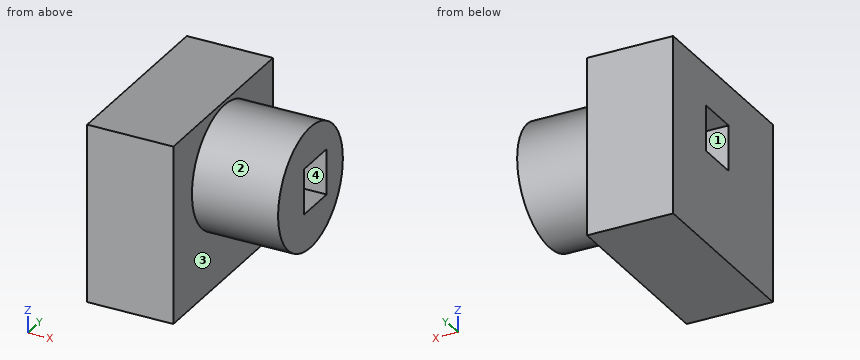
```python
from build123d import *

# Parameters (mm, degrees)
F0_W     = 54.889154
F0_H     = 52.407466
F1_DEPTH = 25.4
F2_R     = 17.820704
F3_DEPTH = 25.4
F4_W     = 12.562469
F4_H     = 13.418828
F5_DEPTH = 50.801


with BuildPart() as f1:
    # F0 (on Right) → F1 (new body)
    with BuildSketch(Plane.YZ):
        with Locations((27.444577, -26.203733)):
            Rectangle(F0_W, F0_H)
    extrude(amount=F1_DEPTH)

    # F2 (on face) → F3 (join)
    with BuildSketch(Plane.YZ.offset(25.4)):
        with Locations((28.055245, -18.92175)):
            Circle(F2_R)
    extrude(amount=F3_DEPTH)

    # F4 (on face) → F5 (cut, through all)
    with BuildSketch(Plane.YZ.offset(50.8)):
        with Locations((30.671432, -18.585598)):
            Rectangle(F4_W, F4_H)
    extrude(amount=-F5_DEPTH, mode=Mode.SUBTRACT)


solid = f1.part
```
Input: part model. Units: mm. Frame: model coordinates. Face numbers are marked on the shaded views. Round coordinates to 2 decimals unless told otherwise and drop trailing zeros. Order: outer loops, then holes, each group sorted by start corner. A loop starts at its lowest first (then second) coordinate and runs counter-clockwise, first axis right, second up. Notation, with made-up numbers: (34, 40.5) - (85, 40.5) arc R23 cw to (85, 77.5) - close; hole circle Ø11 at (45, 57). An arc over 180 degrees is marked (long way). Answer in a Markdown table with one row per item.
Item 1: Section query D-D (z = -34.5). Return the cut outline in (x, y).
Model answer:
| item | result |
|---|---|
| outline | (0, 0) - (25.4, 0) - (25.4, 19.4) - (50.8, 19.4) - (50.8, 36.71) - (25.4, 36.71) - (25.4, 54.89) - (0, 54.89) - close |
Item 2: Pin query (flat end, axial travel): pin 1 (1.5 mm diameter, centred on y = 16, z = -42.5, fed in from +X); pin 2 (10 mm diameter, centred on x = 16, y = 13.5, fed in from +Z); pin 3 (1 mm diameter, centred on x = 36.5, y = 27.5, fed in from -Z); pin 4 (6 mm diameter, centred on x = 40.5, y = 12.5, fed in from +Z). Return the tip coordinate at first contact, or that it passes through.
Model answer:
| item | result |
|---|---|
| pin 1 | stops at x = 25.4 |
| pin 2 | stops at z = 0 |
| pin 3 | stops at z = -36.74 |
| pin 4 | stops at z = -6.27 |
Item 3: Section query A-A (x = 22). Return the cut outline in (y, z), then the cut area to 3 significant figures.
Model answer:
| item | result |
|---|---|
| outline | (0, -52.41) - (54.89, -52.41) - (54.89, 0) - (0, 0) - close; hole (24.39, -25.3) - (36.95, -25.3) - (36.95, -11.88) - (24.39, -11.88) - close |
| area | 2,710 mm² |
Item 4: Line query: line 1 (Z direction, x = 11, y = 28); line 2 (Y direction, x = 32.5, z = -18.5); line 3 (X direction, y = 51.5, z = -14). Output: solid intervals per line, ascending.
Model answer:
| item | result |
|---|---|
| line 1 | z = -52.41 to -25.3, -11.88 to 0 |
| line 2 | y = 10.24 to 24.39, 36.95 to 45.87 |
| line 3 | x = 0 to 25.4 |
Item 5: Section query B-B (z = -15). Return the cut outline in (x, y), then the cut area to 3 significant figures.
Model answer:
| item | result |
|---|---|
| outline | (0, 0) - (25.4, 0) - (25.4, 10.67) - (50.8, 10.67) - (50.8, 24.39) - (0, 24.39) - close; (0, 36.95) - (50.8, 36.95) - (50.8, 45.44) - (25.4, 45.44) - (25.4, 54.89) - (0, 54.89) - close |
| area | 1,640 mm² |
Item 6: Mould query, pull axis Y, two halves, no side actions, for the marked faces 1, 2, 3 and 4. Classes: released by +Y, released by -Y, zero draft, split by the parting line, or undercut.
Model answer:
| item | result |
|---|---|
| face 1 | undercut |
| face 2 | split by the parting line |
| face 3 | zero draft |
| face 4 | undercut |
Item 7: Section query C-C (y = 41). Return the cut outline in (x, z), then the cut area to 3 significant figures.
Model answer:
| item | result |
|---|---|
| outline | (0, -52.41) - (25.4, -52.41) - (25.4, -31.17) - (50.8, -31.17) - (50.8, -6.67) - (25.4, -6.67) - (25.4, 0) - (0, 0) - close |
| area | 1,950 mm² |
